Model file for the job. Use its own axes, mm. Face numbers are marked on the shaded views. A direction names the side the tool comes from. Round coordinates to 2 decimals unless told otherwise and drop trailing zeros. Loops run counter-clockwise (first coordinate to the right, second up) from the corner with the lowest first, then second, coordinate; pieces in that order, holes last. Notation, with made-up numbers: (74.5, 72) -> (123.5, 72) arc R31 ccw to (123.5, 108) -> close; hole circle Ø10 at (47, 14.25). An arc over 180 degrees is marked (long way). Use a Markdown table: item, result. Add a question column.
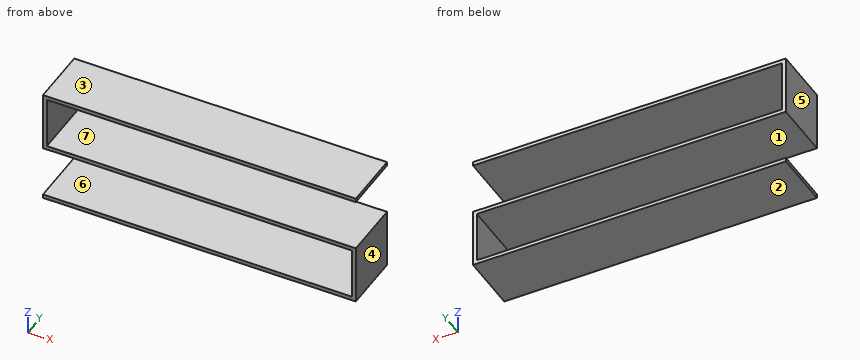
```python
from build123d import *

# Parameters (mm, degrees)
F0_W     = 1524
F0_H     = 285.75
F1_DEPTH = 19.05
F2_W     = 19.05
F2_H     = 285.75
F3_DEPTH = 254
F4_W     = 1504.95
F4_H     = 285.75
F4_W_2   = 19.05
F5_DEPTH = 19.05
F6_W     = 19.05
F6_H     = 285.75
F7_DEPTH = 254
F8_W     = 1504.95
F8_H     = 285.75
F8_W_2   = 19.05
F9_DEPTH = 19.05


with BuildPart() as f1:
    # F0 (on Top) → F1 (new body)
    with BuildSketch(Plane.XY):
        with Locations((186.574653, -79.114271)):
            Rectangle(F0_W, F0_H)
    extrude(amount=F1_DEPTH)

    # F2 (on face) → F3 (join)
    with BuildSketch(Plane(origin=(0, 0, 0), x_dir=(1, 0, 0), z_dir=(0, 0, -1))):
        with Locations((-565.900347, 79.114271)):
            Rectangle(F2_W, F2_H)
    extrude(amount=F3_DEPTH)

    # F4 (on face) → F5 (join)
    with BuildSketch(Plane(origin=(0, 0, -254), x_dir=(1, 0, 0), z_dir=(0, 0, -1))):
        with Locations((196.099653, 79.114271)):
            Rectangle(F4_W, F4_H)
        with Locations((-565.900347, 79.114271)):
            Rectangle(F4_W_2, F4_H)
    extrude(amount=F5_DEPTH)

    # F6 (on face) → F7 (join)
    with BuildSketch(Plane(origin=(0, 0, -273.05), x_dir=(1, 0, 0), z_dir=(0, 0, -1))):
        with Locations((939.049653, 79.114271)):
            Rectangle(F6_W, F6_H)
    extrude(amount=F7_DEPTH)

    # F8 (on face) → F9 (join)
    with BuildSketch(Plane(origin=(0, 0, -527.05), x_dir=(1, 0, 0), z_dir=(0, 0, -1))):
        with Locations((177.049653, 79.114271)):
            Rectangle(F8_W, F8_H)
        with Locations((939.049653, 79.114271)):
            Rectangle(F8_W_2, F8_H)
    extrude(amount=F9_DEPTH)


solid = f1.part
```
1) Cut at C-C on z = -96.5. Write the cut outline in (x, y).
2) Tool access for the marked faces 5, 6 and 7: list every direction of +Z, -Z, +X, -X, +Y, -Y with a clear straight run to the whole face (end or side of a thin tool).
3) Pull direction Z, two halves, no side cores. Call the marked faces 1, 2, 3 and 4: +Z half, -Z half, draft (parallel to the pull), parting line (faces both ways), or undercut.
4) Cut at A-A on x = 399.5. Write the cut outline in (y, z).
5) Wall check: probe 1 along Z at (x, y) = (-417.5, -84); probe 2 along X at (y, z) = (45, -118.5); probe 3 along X at (y, z) = (-101, -353.5). Give the ranges that are in metal, low to high. Write a range as from..to.
6) Pin check, flat tip, straight feed: pin 1 Ø1 at (y, z) = (10.5, -115) entering from +X. Stop position of the tip, or through.
7) Cut at B-B on y = -89. Write the cut outline in (x, z).
Established:
| question | item | result |
|---|---|---|
| 1 | outline | (-575.43, -221.99) -> (-556.38, -221.99) -> (-556.38, 63.76) -> (-575.43, 63.76) -> close |
| 2 | face 5 | +Z, -Z, -X, +Y, -Y |
| 2 | face 6 | -X, +Y, -Y |
| 2 | face 7 | +X, +Y, -Y |
| 3 | face 1 | undercut |
| 3 | face 2 | -Z half |
| 3 | face 3 | +Z half |
| 3 | face 4 | draft |
| 4 | outline | (-221.99, -546.1) -> (63.76, -546.1) -> (63.76, -527.05) -> (-221.99, -527.05) -> close; (-221.99, -273.05) -> (63.76, -273.05) -> (63.76, -254) -> (-221.99, -254) -> close; (-221.99, 0) -> (63.76, 0) -> (63.76, 19.05) -> (-221.99, 19.05) -> close |
| 5 | probe 1 | z = -546.1..-527.05, -273.05..-254, 0..19.05 |
| 5 | probe 2 | x = -575.43..-556.38 |
| 5 | probe 3 | x = 929.52..948.57 |
| 6 | pin 1 | stops at x = -556.38 |
| 7 | outline | (-575.43, -546.1) -> (948.57, -546.1) -> (948.57, -254) -> (-556.38, -254) -> (-556.38, 0) -> (948.57, 0) -> (948.57, 19.05) -> (-575.43, 19.05) -> (-575.43, -273.05) -> (929.52, -273.05) -> (929.52, -527.05) -> (-575.43, -527.05) -> close |
